Geometry: see drawing. Coordinates: mm, zero at the bounding-box minimum. Coordinates: 2 decimals unless noted, no trailing zeros. Write each loop counter-clockwise with the first axis right and the second up, starting at its lowest first coordinate (ties: lowest second). Pieces come first, ordered by that corner, then holes. Notation, with made-up numbers: (-34.75, 17) - (-20.75, 17) arc R8 ccw to (-20.75, 22) - close; hole circle Ø3 at (77.25, 8.5). An arc over 180 degrees is marked (long way). Use CSV: the item, a comma, the result in double quotes.
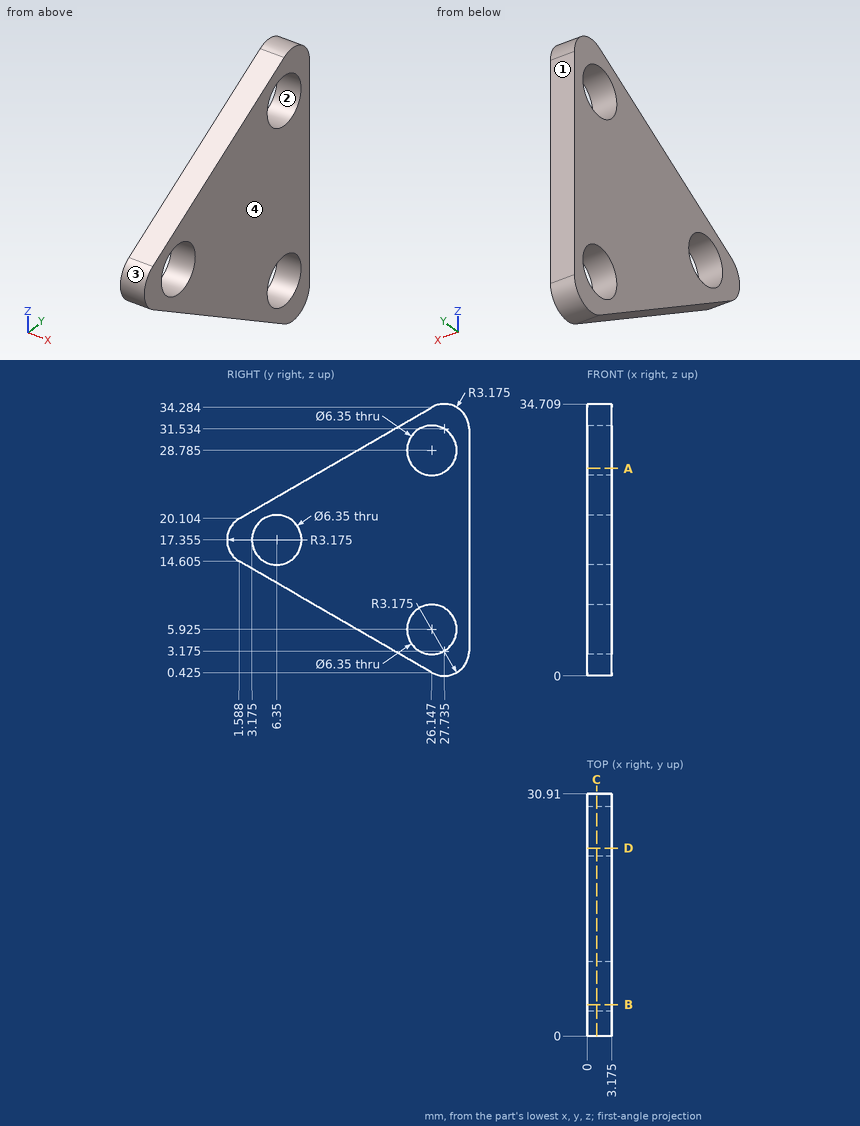
(1) Cut plane A-A on z = 26.5. Return loops of the section in (x, y) (1 decimal).
Check values:
outline,"(0, 12.7) - (3.2, 12.7) - (3.2, 23.9) - (0, 23.9) - close; (0, 28.4) - (3.2, 28.4) - (3.2, 30.9) - (0, 30.9) - close"
(2) Pin query (flat end, axial travel): pin 1 Ø8 at (y, z) = (8.5, 25) entering from +X (3 decimals); pin 2 Ø1.5 at (x, z) = (0.5, 24) entering from -Y (1 decimal). Return the tip coordinate at first contact, or that it passes through.
Check values:
pin 1,"x = 3.175"
pin 2,"y = 7"
(3) Draft query along Y for the marked faces 1, 2, 3 and 4. Return one class per face: pulls with the +Y half, pulls with the -Y half, needs draft (parallel to the pull), parting line crosses it, or undercut.
Check values:
face 1,"pulls with the +Y half"
face 2,"undercut"
face 3,"pulls with the -Y half"
face 4,"needs draft"
(4) Cut plane D-D on y = 24. Return loops of the section in (x, z) (1 decimal).
Check values:
outline,"(0, 1.7) - (3.2, 1.7) - (3.2, 3.6) - (0, 3.6) - close; (0, 8.3) - (3.2, 8.3) - (3.2, 26.4) - (0, 26.4) - close; (0, 31.1) - (3.2, 31.1) - (3.2, 33) - (0, 33) - close"
(5) Cut plane B-B on y = 4. Return loops of the section in (x, z) (1 decimal).
Check values:
outline,"(0, 13.2) - (3.2, 13.2) - (3.2, 15.2) - (0, 15.2) - close; (0, 19.5) - (3.2, 19.5) - (3.2, 21.5) - (0, 21.5) - close"
(6) Ray query, probe 1 along Z at (x, y) = (0.9, 5) (1 decimal); probe 2 along Y at (x, z) = (1, 18) (1 decimal); probe 3 along Z at (x, y) = (0.65, 9) (1 decimal). Return the intervals inside material, ascending. Write a range as from..to.
Check values:
probe 1,"12.6..14.5, 20.2..22.1"
probe 2,"0.1..3.2, 9.5..30.9"
probe 3,"10.3..15.6, 19.1..24.4"
(7) Cut plane C-C on x = 1.2. State how many separate pieces and enclosed holes the cut face has, and give its area (3 significant figures).
Check values:
separate pieces,"1"
enclosed holes,"3"
area,"555 mm^2"
